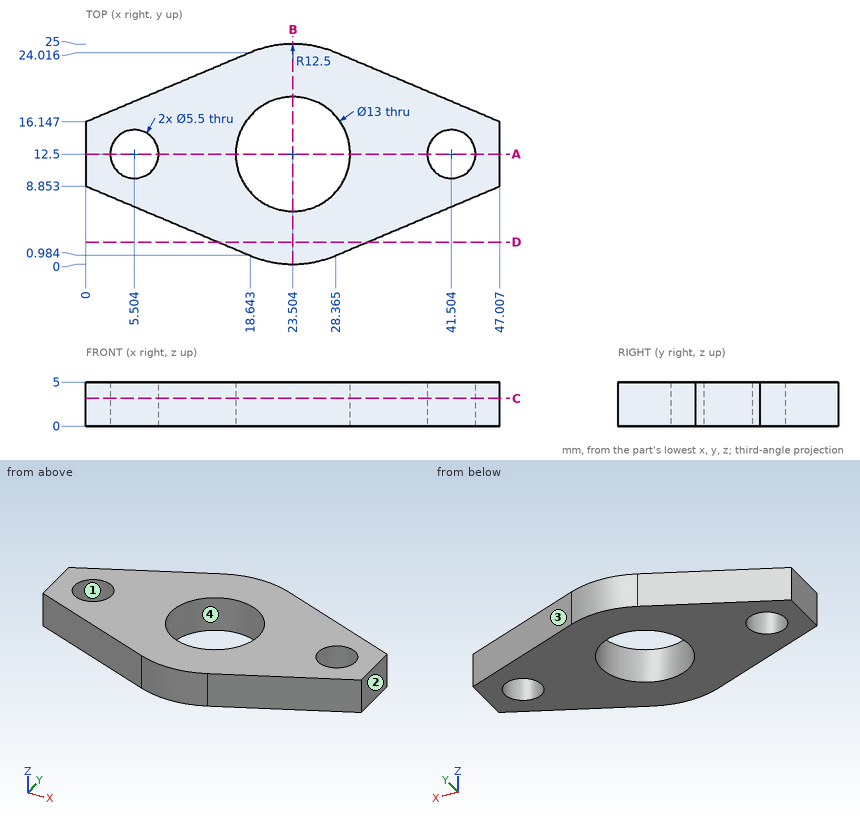
Can you work these out from the drawing? Everything is in mm from the part's minimum corner. Round coordinates to 2 decimals unless told otherwise and drop trailing zeros. Loops run counter-clockwise (first coordinate to the right, second up) from the corner with the lowest first, then second, coordinate; pieces in that order, holes last. Notation, with made-up numbers: (51.25, -15) -> (59.25, -15) arc R19 ccw to (59.25, 18) -> close; hole circle Ø1 at (39.25, 55). An arc over 180 degrees is marked (long way). Put each result on its own line as item: value.
Q1. Please list where these lines run through material, in increasing order: line 1 (X direction, y = 13.5, z = 3.7) (1 decimal); line 2 (X direction, y = 11.25, z = 4.1) (1 decimal); line 3 (Y direction, x = 21, z = 0.85). Write a range as from..to.
Checks:
line 1: 0..2.9, 8.1..17.1, 29.9..38.9, 44.1..47
line 2: 0..3.1, 8..17.1, 29.9..39.1, 44..47
line 3: 0.25..6.5, 18.5..24.75
Q2. I want a section at B-B on x = 23.5. Write out the boundary of the cut face in (y, z).
Checks:
outline: (0, 0) -> (6, 0) -> (6, 5) -> (0, 5) -> close; (19, 0) -> (25, 0) -> (25, 5) -> (19, 5) -> close
Q3. For pin 1 Ø5 at (x, y) = (41.5, 12.5) entering from +Z; pin 2 Ø1 at (y, z) = (12.5, 4) entering from -X; pin 3 Ø3 at (x, z) = (31.5, 4) entering from +Y (1 decimal), each with a flat end and sliding along its axis, tell me the tip position at first contact or that it passes through.
Checks:
pin 1: through
pin 2: x = 0
pin 3: y = 23.3
Q4. I want a section at C-C on z = 3.15. Give the number of separate pieces and of enclosed holes in the cut face, and give its area (3 significant figures).
Checks:
separate pieces: 1
enclosed holes: 3
area: 622 mm2
Q5. I want a section at A-A on y = 12.5. Write out the boundary of the cut face in (x, z).
Checks:
outline: (0, 0) -> (2.75, 0) -> (2.75, 5) -> (0, 5) -> close; (8.25, 0) -> (17, 0) -> (17, 5) -> (8.25, 5) -> close; (30, 0) -> (38.75, 0) -> (38.75, 5) -> (30, 5) -> close; (44.25, 0) -> (47.01, 0) -> (47.01, 5) -> (44.25, 5) -> close
Q6. I want a section at D-D on y = 2.5. Write out the boundary of the cut face in (x, z).
Checks:
outline: (15.05, 0) -> (31.96, 0) -> (31.96, 5) -> (15.05, 5) -> close
Q7. Thinking about a two-plate mould opening in Y: for the marked faces 1, 2, 3 and 4, which applies, pulls with the +Y half, pulls with the -Y half, needs draft (parallel to the pull), parting line crosses it, or undercut?
Checks:
face 1: undercut
face 2: needs draft
face 3: pulls with the +Y half
face 4: undercut
